from build123d import *

# Parameters (mm, degrees)
SKETCH1_R           = 1.75
BOSS_EXTRUDE1_DEPTH = 2


with BuildPart() as part:
    # Sketch1 → Boss-Extrude1 (new body)
    with BuildSketch(Plane.XY):
        with BuildLine():
            Line((-19.75, 7.1), (-19.75, -7.1))
            ThreePointArc((-19.75, -7.1), (-19.457106781, -7.807106781), (-18.75, -8.1))
            Line((-18.75, -8.1), (18.75, -8.1))
            ThreePointArc((18.75, -8.1), (19.457106781, -7.807106781), (19.75, -7.1))
            Line((19.75, -7.1), (19.75, 7.1))
            ThreePointArc((19.75, 7.1), (19.457106781, 7.807106781), (18.75, 8.1))
            Line((18.75, 8.1), (-18.75, 8.1))
            ThreePointArc((-18.75, 8.1), (-19.457106781, 7.807106781), (-19.75, 7.1))
        make_face()
        with Locations(Location((-16.25, 5.1, 0), (0, 0, 180))):
            Circle(SKETCH1_R, mode=Mode.SUBTRACT)
        with Locations(Location((2.5, 5.1, 0), (0, 0, 180))):
            Circle(SKETCH1_R, mode=Mode.SUBTRACT)
        with BuildLine():
            Line((7.25, 5.1), (10.75, 5.1))
            ThreePointArc((10.75, 5.1), (11.457106781, 4.807106781), (11.75, 4.1))
            Line((11.75, 4.1), (11.75, -2.9))
            ThreePointArc((11.75, -2.9), (11.457106781, -3.607106781), (10.75, -3.9))
            Line((10.75, -3.9), (7.25, -3.9))
            ThreePointArc((7.25, -3.9), (6.542893219, -3.607106781), (6.25, -2.9))
            Line((6.25, -2.9), (6.25, 4.1))
            ThreePointArc((6.25, 4.1), (6.542893219, 4.807106781), (7.25, 5.1))
        make_face(mode=Mode.SUBTRACT)
        with BuildLine():
            Line((-12.95, 2.1), (-0.95, 2.1))
            ThreePointArc((-0.95, 2.1), (-0.242893219, 1.807106781), (0.05, 1.1))
            Line((0.05, 1.1), (0.05, -2.4))
            ThreePointArc((0.05, -2.4), (-0.242893219, -3.107106781), (-0.95, -3.4))
            Line((-0.95, -3.4), (-12.95, -3.4))
            ThreePointArc((-12.95, -3.4), (-13.657106781, -3.107106781), (-13.95, -2.4))
            Line((-13.95, -2.4), (-13.95, 1.1))
            ThreePointArc((-13.95, 1.1), (-13.657106781, 1.807106781), (-12.95, 2.1))
        make_face(mode=Mode.SUBTRACT)
    extrude(amount=-BOSS_EXTRUDE1_DEPTH)


solid = part.part
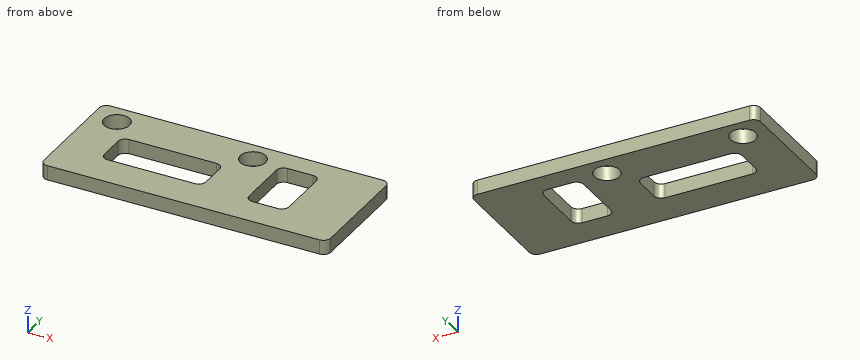
Verification items for the finished model (mm, model axes). Coordinates: 2 decimals unless noted, no trailing zeros. Loops run counter-clockwise (first coordinate to the right, second up) from the corner with the lowest first, then second, coordinate; pieces in that order, holes last. Notation, with made-up numbers: M 64,-20 L 99,-20 A28 ccw 99,10 Z; hole C -9,20 d3. An arc over 180 degrees is marked long. One line per item, written item: value.
1. Section check B-B on z = -1.3. Record the cut outline in (x, y), plus the area to 3 significant figures.
Answers follow:
outline: M -19.75,-7.1 A1 ccw -18.75,-8.1 L 18.75,-8.1 A1 ccw 19.75,-7.1 L 19.75,7.1 A1 ccw 18.75,8.1 L -18.75,8.1 A1 ccw -19.75,7.1 Z; hole C -16.25,5.1 d3.5; hole M -13.95,-2.4 A1 ccw -12.95,-3.4 L -0.95,-3.4 A1 ccw 0.05,-2.4 L 0.05,1.1 A1 ccw -0.95,2.1 L -12.95,2.1 A1 ccw -13.95,1.1 Z; hole C 2.5,5.1 d3.5; hole M 6.25,-2.9 A1 ccw 7.25,-3.9 L 10.75,-3.9 A1 ccw 11.75,-2.9 L 11.75,4.1 A1 ccw 10.75,5.1 L 7.25,5.1 A1 ccw 6.25,4.1 Z
area: 495 mm^2
2. Material ranges on line 1 along X through (y, z) = (-1.75, -0.45); line 2 along X through (y, z) = (-2.5, -1.35); line 3 along Y through (x, z) = (10, -1.25), recorded low to high. Write a range as from..to.
Answers follow:
line 1: -19.75..-13.95, 0.05..6.25, 11.75..19.75
line 2: -19.75..-13.94, 0.04..6.25, 11.75..19.75
line 3: -8.1..-3.9, 5.1..8.1
3. Section check C-C on x = 8.5. Record the cut outline in (y, z), plus the area to 3 significant figures.
Answers follow:
outline: M -8.1,-2 L -3.9,-2 L -3.9,0 L -8.1,0 Z; M 5.1,-2 L 8.1,-2 L 8.1,0 L 5.1,0 Z
area: 14.4 mm^2
4. Section check A-A on x = 2.5. Record the cut outline in (y, z), plus the area to 3 significant figures.
Answers follow:
outline: M -8.1,-2 L 3.35,-2 L 3.35,0 L -8.1,0 Z; M 6.85,-2 L 8.1,-2 L 8.1,0 L 6.85,0 Z
area: 25.4 mm^2
